Work out the finished part from the listing and answer in its coordinate system (mm). Coordinates: 2 decimals unless noted, no trailing zeros. Write each loop counter-clockwise with the first axis right and the second up, starting at its lowest first coordinate (ties: lowest second). Pieces come first, ordered by that corner, then holes. Notation, with made-up numbers: (-33.75, 73) -> (-19.75, 73) arc R13 cw to (-19.75, 95) -> close; hole circle Ø1 at (23.5, 81). An arc over 180 degrees is marked (long way). Write each question's results on one line, items separated by ' | '. Start each with the question number.
Autodesk Inventor part; units mm, degrees
ref_plane "YZ Plane" through (0, 0, 0) normal (1, 0, 0) x (0, 1, 0)
ref_plane "XZ Plane" through (0, 0, 0) normal (0, 1, 0) x (-1, 0, 0)
ref_plane "XY Plane" through (0, 0, 0) normal (0, 0, 1) x (1, 0, 0)
sketch "Sketch1" plane through (0, 0, 0) normal (0, 1, 0) x (-1, 0, 0)
  line L0 (-29.1562, -50.5) -> (-58.3124, 0)
  line L1 (-58.3124, 0) -> (-29.1562, 50.5)
  line L2 (-29.1562, 50.5) -> (29.1562, 50.5)
  line L3 (29.1562, 50.5) -> (58.3124, 0)
  line L4 (58.3124, 0) -> (29.1562, -50.5)
  line L5 (29.1562, -50.5) -> (-29.1562, -50.5)
  point P0 (0, 0)
  point P1 (0, 0)
  dimension "d0" = 101
extrude "Extrusion1" add sketch "Sketch1" along normal mid plane 30.9
properties part number "Hex_Reds" material "Paper"
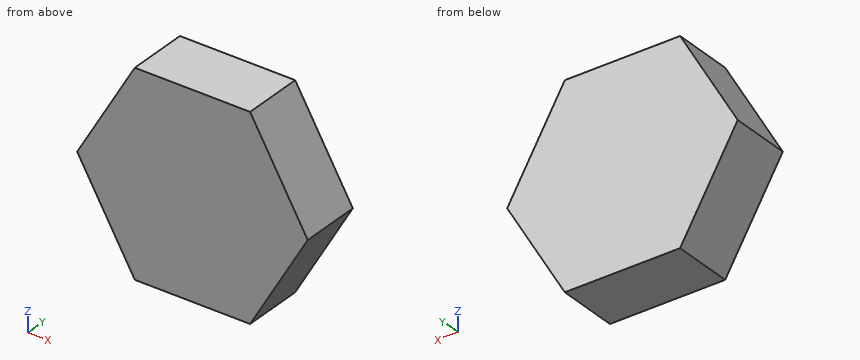
1. Find section B-B on z = 25.5. Give the vertices of the cut face in (x, y), and give its area (3 significant figures).
2. Find the intervals of material crossed by L1, parallel to X at y = 12.5, z = -29.5; L2, parallel to Z at x = -32.5, y = 14; L3, parallel to X at y = -8, z = -26, in increasing order.
3. Given pin 1 Ø8 at (y, z) = (4, 10) entering from +X; pin 2 Ø8 at (y, z) = (-9.5, -8.5) entering from +X; pin 3 Ø6 at (y, z) = (5, -11) entering from +X, each flat-ended and moving along its own axis, determine where each tip first touches the part or whether it passes through.
4. Find section C-C on x = -44. Give the vertices of the cut face in (y, z), and give its area (3 significant figures).
5. Find section A-A on y = -4. Give the vertices of the cut face in (x, z), and give its area (3 significant figures).
Ans:
1) outline: (-43.59, -15.45) -> (43.59, -15.45) -> (43.59, 15.45) -> (-43.59, 15.45) -> close | area: 2,690 mm²
2) L1: x = -41.28 to 41.28 | L2: z = -44.71 to 44.71 | L3: x = -43.3 to 43.3
3) pin 1: stops at x = 54.85 | pin 2: stops at x = 55.71 | pin 3: stops at x = 53.69
4) outline: (-15.45, -24.79) -> (15.45, -24.79) -> (15.45, 24.79) -> (-15.45, 24.79) -> close | area: 1,530 mm²
5) outline: (-58.31, 0) -> (-29.16, -50.5) -> (29.16, -50.5) -> (58.31, 0) -> (29.16, 50.5) -> (-29.16, 50.5) -> close | area: 8,830 mm²
